CAD build for the part. Positions are in the model's coordinates, mm. A direction names the side the tool comes from. Coordinates: 2 decimals unless noted, no trailing zeros. Loops run counter-clockwise (first coordinate to the right, second up) from the corner with the lowest first, then second, coordinate; pieces in that order, holes last. Notation, with made-up numbers: (4, -10.5) -> (11, -10.5) arc R27 ccw to (11, 25.5) -> close; hole circle Ø6 at (37.25, 45). An arc over 180 degrees is marked (long way). Write item = value, one per line. Start each with the question number.
(1) Flat gauge pins, fed straight in: P1, Ø4, axis at y = 17.5, z = -24, coming from the +X side; P2, Ø0.6, axis at x = -61.5, z = 1, coming from the +Y side; P3, Ø2, axis at x = -55, y = 19, coming from the +Z side; P4, Ø4, axis at x = -39.5, y = 24.5, coming from the +Z side. Where does each tip first touch, or does it go through?
(2) Tool access for faces 5 (the face through (-46, 20, -32)), 6 (the face through (-34.7, 31.9, 0)), 7 (the face through (-56.1, 31.9, 0)): list every direction of +Z, -Z, +X, -X, +Y, -Y with a clear straight run to the whole face (end or side of a thin tool).
(3) Band-saw the part on D-D (y = 25.5). Write the cut outline in (x, z), and give its area (3 significant figures).
(4) Band-saw the part on B-B (x = -37.5). Write the cut outline in (y, z).
(5) Drill centre lines: line 1 (Y direction, x = -29.5, z = -15); line 2 (Y direction, x = -56, z = -17); line 3 (X direction, y = 28.25, z = -23). Where is each one in solid material? Low to high. Write a range as from..to.
(6) Band-saw the part on C-C (z = -29.5). Write the cut outline in (x, y).
(7) Pull direction X, two halves, no side cores. Call faces 1 (the face through (-61.088, 25, -15)), 2 (the face through (-61.34, 18.29, -26.55)), 3 (the face through (-61.588, 25, -15)), 4 (the face through (-46, 31.567, -11)): +X half, -X half, draft (parallel to the pull), parting line (faces both ways), or undercut.
(8) Band-saw the part on A-A (z = -17). Write the cut outline in (x, y), and give its area (3 significant figures).
```python
from build123d import *

# Parameters (mm, degrees)
ESQUISSE1_W             = 32.5
ESQUISSE1_H             = 17.5
ESQUISSE1_W_2           = 31.5
ESQUISSE1_H_2           = 16.5
BASE_EXTRUSION_DEPTH    = 32
ESQUISSE3_W             = 0.5
ESQUISSE3_H             = 17.5
BOSS_EXTRU_1_DEPTH      = 32.5
ENL_V_MAT_EXTRU_1_DEPTH = 57.042915794
ESQUISSE5_W             = 1
ESQUISSE5_H             = 0.5
ESQUISSE5_W_2           = 0.5
ESQUISSE5_H_2           = 1
BOSS_EXTRU_2_DEPTH      = 2
ENL_V_MAT_EXTRU_2_DEPTH = 35.693670075
EXTRUSION2_DEPTH        = 32.5


with BuildPart() as part:
    # Esquisse1 → Base-Extrusion (new body)
    with BuildSketch(Plane.XY):
        with Locations((-45.33773679, 23.317248255)):
            Rectangle(ESQUISSE1_W, ESQUISSE1_H)
        with Locations((-45.33773679, 23.317248255)):
            Rectangle(ESQUISSE1_W_2, ESQUISSE1_H_2, mode=Mode.SUBTRACT)
    extrude(amount=-BASE_EXTRUSION_DEPTH)

    # Esquisse3 → Boss.-Extru.1 (add)
    with BuildSketch(Plane.ZY.offset(61.58773679)):
        with Locations((-32.25, 23.317248255)):
            Rectangle(ESQUISSE3_W, ESQUISSE3_H)
    extrude(amount=-BOSS_EXTRU_1_DEPTH)

    # Esquisse4 → Enlèv. mat.-Extru.1 (cut, through all)
    with BuildSketch(Plane.ZY.offset(61.58773679)):
        with BuildLine():
            Line((-23.4, 15.067248255), (0.817293984, 15.067248255))
            Line((0.817293984, 15.067248255), (0.817293984, 21.367248255))
            Line((0.817293984, 21.367248255), (-23.4, 21.367248255))
            ThreePointArc((-23.4, 21.367248255), (-26.55, 18.217248255), (-23.4, 15.067248255))
        make_face()
    extrude(amount=-ENL_V_MAT_EXTRU_1_DEPTH, mode=Mode.SUBTRACT)

    # Esquisse5 → Boss.-Extru.2 (add)
    with BuildSketch(Plane.XY):
        with Locations((-45.33773679, 14.817248255)):
            Rectangle(ESQUISSE5_W, ESQUISSE5_H)
        with Locations((-29.33773679, 23.317248255)):
            Rectangle(ESQUISSE5_W_2, ESQUISSE5_H_2)
        with Locations((-45.33773679, 31.817248255)):
            Rectangle(ESQUISSE5_W, ESQUISSE5_H)
        with Locations((-61.33773679, 23.317248255)):
            Rectangle(ESQUISSE5_W_2, ESQUISSE5_H_2)
    extrude(amount=BOSS_EXTRU_2_DEPTH)

    # Esquisse6 → Enlèv. mat.-Extru.2 (cut)
    with BuildSketch(Plane.ZY.offset(61.58773679)):
        Polygon((-41.526935662, 26.437225615), (-29.203507462, 38.760653816), (-23.505050951, 33.062197305), (-35.828479151, 20.738769104), align=None)
    extrude(amount=-ENL_V_MAT_EXTRU_2_DEPTH, mode=Mode.SUBTRACT)

    # Esquisse7 → Extrusion2 (add)
    with BuildSketch(Plane.ZY.offset(61.58773679)):
        Polygon((-32.5, 24.067248255), (-24.5, 32.067248255), (-25.207106781, 32.067248255), (-32.5, 24.774355036), align=None)
    extrude(amount=-EXTRUSION2_DEPTH)


solid = part.part
```
Findings below:
q1.P1 = through
q1.P2 = 23.82
q1.P3 = -32
q1.P4 = -30.07
q2.face_5 = +Z
q2.face_6 = +Z, +X, +Y
q2.face_7 = +Z, -X, +Y
q3.outline = (-61.59, -31.77) -> (-29.09, -31.77) -> (-29.09, 0) -> (-29.59, 0) -> (-29.59, -31.07) -> (-61.09, -31.07) -> (-61.09, 0) -> (-61.59, 0) -> close
q3.area = 54.0 mm²
q4.outline = (14.57, -32.5) -> (24.77, -32.5) -> (32.07, -25.21) -> (32.07, 0) -> (31.57, 0) -> (31.57, -25) -> (24.57, -32) -> (15.07, -32) -> (15.07, 0) -> (14.57, 0) -> close
q5.line_1 = 14.57..15.07, 21.37..32.07
q5.line_2 = 14.57..15.07, 31.57..32.07
q5.line_3 = -61.59..-61.09, -29.59..-29.09
q6.outline = (-61.59, 14.57) -> (-29.09, 14.57) -> (-29.09, 27.77) -> (-61.59, 27.77) -> close; hole (-61.09, 15.07) -> (-29.59, 15.07) -> (-29.59, 27.07) -> (-61.09, 27.07) -> close
q7.face_1 = undercut
q7.face_2 = draft
q7.face_3 = -X half
q7.face_4 = undercut
q8.outline = (-61.59, 14.57) -> (-29.09, 14.57) -> (-29.09, 15.07) -> (-61.59, 15.07) -> close; (-61.59, 21.37) -> (-61.09, 21.37) -> (-61.09, 31.57) -> (-29.59, 31.57) -> (-29.59, 21.37) -> (-29.09, 21.37) -> (-29.09, 32.07) -> (-61.59, 32.07) -> close
q8.area = 42.7 mm²
